```python
from build123d import *

# Parameters (mm, degrees)
SKETCH_1_W      = 35
SKETCH_1_H      = 130
SKETCH_1_R      = 1.6
SKETCH_1_W_2    = 3
SKETCH_1_H_2    = 18
SKETCH_1_W_3    = 10
SKETCH_1_H_3    = 33
EXTRUDE_1_DEPTH = 2
FILLET_1_R      = 2


with BuildPart() as part:
    # 草图1 → 凸台-拉伸1 (new body)
    with BuildSketch(Plane(origin=(0, 0, 0), x_dir=(1, 0, 0), z_dir=(0, 1, 0))):
        with Locations((-17.5, 0)):
            Rectangle(SKETCH_1_W, SKETCH_1_H)
        with Locations(Location((-10, 60, 0), (0, 0, 270))):
            Circle(SKETCH_1_R, mode=Mode.SUBTRACT)
        with Locations(Location((-10, 40, 0), (0, 0, 270))):
            Circle(SKETCH_1_R, mode=Mode.SUBTRACT)
        with Locations(Location((-10, 20, 0), (0, 0, 270))):
            Circle(SKETCH_1_R, mode=Mode.SUBTRACT)
        with Locations(Location((-10, 0, 0), (0, 0, 270))):
            Circle(SKETCH_1_R, mode=Mode.SUBTRACT)
        with Locations(Location((-10, -20, 0), (0, 0, 270))):
            Circle(SKETCH_1_R, mode=Mode.SUBTRACT)
        with Locations((-29.5, 50)):
            Rectangle(SKETCH_1_W_2, SKETCH_1_H_2, mode=Mode.SUBTRACT)
        with Locations((-21.5, 50)):
            Rectangle(SKETCH_1_W_2, SKETCH_1_H_2, mode=Mode.SUBTRACT)
        with Locations((-29.5, 25)):
            Rectangle(SKETCH_1_W_2, SKETCH_1_H_2, mode=Mode.SUBTRACT)
        with Locations((-29.5, 0)):
            Rectangle(SKETCH_1_W_2, SKETCH_1_H_2, mode=Mode.SUBTRACT)
        with Locations((-29.5, -25)):
            Rectangle(SKETCH_1_W_2, SKETCH_1_H_2, mode=Mode.SUBTRACT)
        with Locations((-29.5, -50)):
            Rectangle(SKETCH_1_W_2, SKETCH_1_H_2, mode=Mode.SUBTRACT)
        with Locations((-21.5, 25)):
            Rectangle(SKETCH_1_W_2, SKETCH_1_H_2, mode=Mode.SUBTRACT)
        with Locations((-21.5, 0)):
            Rectangle(SKETCH_1_W_2, SKETCH_1_H_2, mode=Mode.SUBTRACT)
        with Locations((-21.5, -25)):
            Rectangle(SKETCH_1_W_2, SKETCH_1_H_2, mode=Mode.SUBTRACT)
        with Locations((-21.5, -50)):
            Rectangle(SKETCH_1_W_2, SKETCH_1_H_2, mode=Mode.SUBTRACT)
        with Locations((-10, -42.5)):
            Rectangle(SKETCH_1_W_3, SKETCH_1_H_3, mode=Mode.SUBTRACT)
    extrude(amount=EXTRUDE_1_DEPTH)

    # 圆角1
    fillet_1_edges = [part.edges().sort_by_distance(p)[0] for p in [
        (0, 1, 65),
        (-35, 1, 65),
        (-35, 1, -65),
        (0, 1, -65),
    ]]
    fillet(fillet_1_edges, radius=FILLET_1_R)


solid = part.part
```
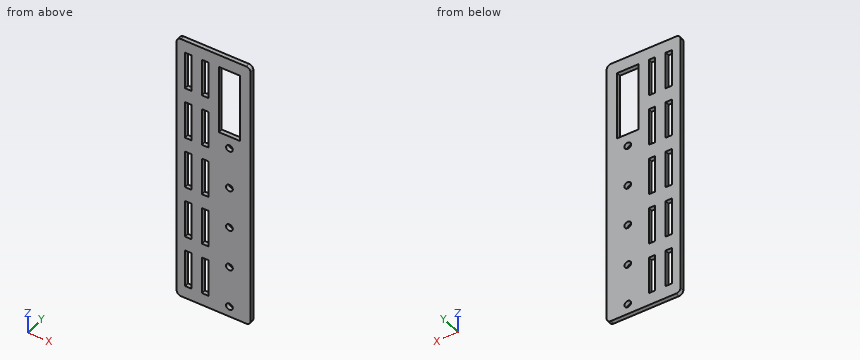
Work out the finished part from the listing and answer in its coordinate system (mm). Round coordinates to 2 decimals unless told otherwise and drop trailing zeros. Loops run counter-clockwise (first coordinate to the right, second up) from the corner with the lowest first, then second, coordinate; pieces in that order, holes last.
(1) Find the intervals of material crossed by L1, parallel to X at y = 0.8, z = 20; L2, parallel to X at y = 1.6, z = 56; L3, parallel to X at y = 0.3, z = -4, in increasing order.
Computed values:
L1: x = -35 to -31, -28 to -23, -20 to -11.6, -8.4 to 0
L2: x = -35 to -31, -28 to -23, -20 to -15, -5 to 0
L3: x = -35 to -31, -28 to -23, -20 to 0
(2) The part is cut by section D-D, the plane z = -7. Give the vertices of the cut face in (x, y).
Computed values:
outline: (-35, 0) - (-31, 0) - (-31, 2) - (-35, 2) - close; (-28, 0) - (-23, 0) - (-23, 2) - (-28, 2) - close; (-20, 0) - (0, 0) - (0, 2) - (-20, 2) - close
(3) The part is cut by section C-C, the plane z = 20. Give the vertices of the cut face in (x, y), and give its area (3 significant figures).
Computed values:
outline: (-35, 0) - (-31, 0) - (-31, 2) - (-35, 2) - close; (-28, 0) - (-23, 0) - (-23, 2) - (-28, 2) - close; (-20, 0) - (-11.6, 0) - (-11.6, 2) - (-20, 2) - close; (-8.4, 0) - (0, 0) - (0, 2) - (-8.4, 2) - close
area: 51.6 mm2
(4) The part is cut by section A-A, the plane z = 36.5. Give the vertices of the cut face in (x, y), and give its area (3 significant figures).
Computed values:
outline: (-35, 0) - (-15, 0) - (-15, 2) - (-35, 2) - close; (-5, 0) - (0, 0) - (0, 2) - (-5, 2) - close
area: 50.0 mm2
(5) The part is cut by section B-B, the plane x = -6.5. Give the vertices of the cut face in (y, z).
Computed values:
outline: (0, -65) - (2, -65) - (2, 26) - (0, 26) - close; (0, 59) - (2, 59) - (2, 65) - (0, 65) - close
